from build123d import *

# Parameters (mm, degrees)
F1_DEPTH  = 38.1
F3_DEPTH  = 19.05
F5_DEPTH  = 19.05
F6_W      = 38.1
F6_H      = 19.05
F7_DEPTH  = 38.1
F8_W      = 19.05
F8_H      = 3.175
F9_DEPTH  = 38.1
F10_W     = 19.05
F10_H     = 3.175
F11_DEPTH = 38.1
F12_W     = 38.1
F12_H     = 19.05
F13_DEPTH = 38.1


with BuildPart() as f1:
    # F0 (on Front) → F1 (new body)
    with BuildSketch(Plane.XZ):
        Polygon((396.875, 0), (0, 0), (3.333318, -38.1), (393.541682, -38.1), align=None)
    extrude(amount=F1_DEPTH)

    # F2 (on face) → F3 (cut)
    with BuildSketch(Plane.XZ.offset(38.1)):
        Polygon((396.875, 0), (358.629464, 0), (355.296146, -38.1), (393.541682, -38.1), align=None)
    extrude(amount=-F3_DEPTH, mode=Mode.SUBTRACT)

    # F4 (on face) → F5 (cut)
    with BuildSketch(Plane.XZ.offset(38.1)):
        Polygon((41.578854, -38.1), (38.245536, 0), (0, 0), (3.333318, -38.1), align=None)
    extrude(amount=-F5_DEPTH, mode=Mode.SUBTRACT)

    # F6 (on face) → F7 (cut)
    with BuildSketch(Plane.XZ.offset(38.1)):
        with Locations((295.275, -9.525)):
            Rectangle(F6_W, F6_H)
    extrude(amount=-F7_DEPTH, mode=Mode.SUBTRACT)

    # F8 (on face) → F9 (cut)
    with BuildSketch(Plane.XZ.offset(38.1)):
        with Locations((60.483318, -36.5125)):
            Rectangle(F8_W, F8_H)
    extrude(amount=-F9_DEPTH, mode=Mode.SUBTRACT)

    # F10 (on face) → F11 (cut)
    with BuildSketch(Plane.XZ.offset(38.1)):
        with Locations((336.391682, -36.5125)):
            Rectangle(F10_W, F10_H)
    extrude(amount=-F11_DEPTH, mode=Mode.SUBTRACT)

    # F12 (on face) → F13 (cut)
    with BuildSketch(Plane.XZ.offset(38.1)):
        with Locations((101.6, -9.525)):
            Rectangle(F12_W, F12_H)
    extrude(amount=-F13_DEPTH, mode=Mode.SUBTRACT)


solid = f1.part
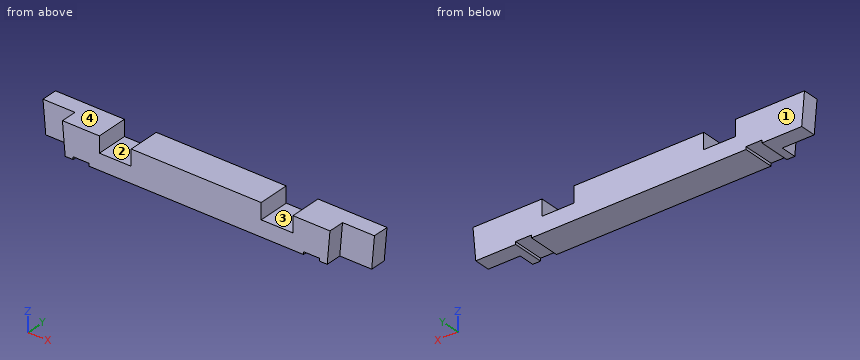
Check sheet for the modelled part. Datum: model origin and axes. Units: mm. Face numbers are marked on the shaded views. A direction names the side the tool comes from. Coordinates: 2 decimals unless noted, no trailing zeros. Write each loop counter-clockwise with the first axis right and the second up, starting at its lowest first coordinate (ties: lowest second). Pieces come first, ordered by that corner, then holes.
Item 1: Scan lines: probe 1 along X at (y, z) = (-19, -18) (3 decimals); probe 2 along X at (y, z) = (-15.5, -17) (3 decimals); probe 3 along Z at (x, y) = (292.5, -11). Record each from-to range of solid material in increasing order.
Numbers:
probe 1: x = 1.575 to 82.55, 120.65 to 276.225, 314.325 to 395.3
probe 2: x = 1.487 to 82.55, 120.65 to 276.225, 314.325 to 395.388
probe 3: z = -38.1 to -19.05
Item 2: Cross-section at B-B on z = -15. Record the boundary of the cut face in (x, y) (3 decimals), then the cut area to 3 significant figures.
Numbers:
outline: (1.312, -19.05) - (39.558, -19.05) - (39.558, -38.1) - (82.55, -38.1) - (82.55, 0) - (1.312, 0) - close; (120.65, -38.1) - (276.225, -38.1) - (276.225, 0) - (120.65, 0) - close; (314.325, -38.1) - (357.317, -38.1) - (357.317, -19.05) - (395.563, -19.05) - (395.563, 0) - (314.325, 0) - close
area: 10,700 mm2
Item 3: Depth check by flat-ended pin: pin 1 Ø1.5 at (y, z) = (-9.5, -6) entering from -X; pin 2 Ø2.5 at (y, z) = (-25.5, -36) entering from +X; pin 3 Ø6 at (y, z) = (-18.5, -13.5) entering from +X. Enter the tip coordinate at first touch or a pass-through.
Numbers:
pin 1: stops at x = 0.46
pin 2: stops at x = 355.59
pin 3: stops at x = 395.96
Item 4: Cross-section at D-D on x = 339. Record the boundary of the cut face in (y, z) (3 decimals), then the cut area to 3 significant figures.
Numbers:
outline: (-38.1, -34.925) - (0, -34.925) - (0, 0) - (-38.1, 0) - close
area: 1,330 mm2
Item 5: Cross-section at C-C on x = 117. Record the boundary of the cut face in (y, z), then the cut area to 3 significant figures.
Numbers:
outline: (-38.1, -38.1) - (0, -38.1) - (0, -19.05) - (-38.1, -19.05) - close
area: 726 mm2
Item 6: Access from +Z, -Z, +X, -X, +Y, -Y to the whole of each face (thin tool, end or side, straight path). Record for the marked faces 3 and 4.
Numbers:
face 3: +Z, +Y, -Y
face 4: +Z, +X, -X, +Y, -Y
Item 7: Cross-section at A-A on y = -13.5. Record the boundary of the cut face in (x, z) (3 decimals).
Numbers:
outline: (0, 0) - (3.333, -38.1) - (50.958, -38.1) - (50.958, -34.925) - (70.008, -34.925) - (70.008, -38.1) - (326.867, -38.1) - (326.867, -34.925) - (345.917, -34.925) - (345.917, -38.1) - (393.542, -38.1) - (396.875, 0) - (314.325, 0) - (314.325, -19.05) - (276.225, -19.05) - (276.225, 0) - (120.65, 0) - (120.65, -19.05) - (82.55, -19.05) - (82.55, 0) - close
Item 8: Mould release check, pull along X, two halves, no side actions. Record for the marked faces 1 and 2: released by +X, released by -X, zero draft, split by the parting line, or undercut.
Numbers:
face 1: zero draft
face 2: undercut
